Input: part model. Units: mm. Frame: model coordinates. Round coordinates to 2 decimals unless told otherwise and drop trailing zeros. Order: outer loops, then holes, each group sorted by start corner. A loop starts at its lowest first (then second) coordinate and runs counter-clockwise, first axis right, second up. Notation, with made-up numbers: (19.5, -2.75) -> (26.5, -2.75) arc R21 cw to (26.5, 26.25) -> close; hole circle Ø5 at (40, 72). An arc over 180 degrees is marked (long way). Use a Markdown table: item, result.
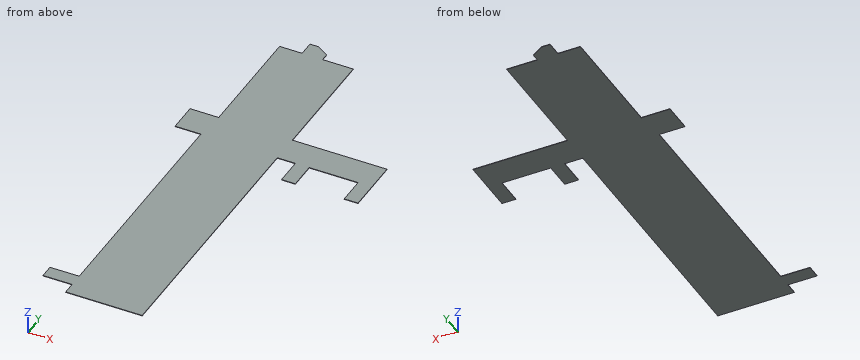
from build123d import *

# Parameters (mm, degrees)
SKETCH_1_W      = 16
SKETCH_1_H      = 30
SKETCH_1_W_2    = 27
SKETCH_1_H_2    = 53
SKETCH_1_W_3    = 60
SKETCH_1_H_3    = 55
SKETCH_1_H_4    = 57.5
SKETCH_1_H_5    = 117
SKETCH_1_H_6    = 117.5
SKETCH_1_W_4    = 125.5
SKETCH_1_H_7    = 60.4
SKETCH_1_H_8    = 230.9
EXTRUDE_1_DEPTH = 1
SKETCH_2_W      = 16
SKETCH_2_H      = 30
EXTRUDE_2_DEPTH = 10


with BuildPart() as part:
    # 草图1 → 拉伸1 (new body)
    with BuildSketch(Plane.XY.offset(42)):
        with Locations((450.5, -369.2)):
            Rectangle(SKETCH_1_W, SKETCH_1_H)
        Polygon((384.5, -354.2), (384.5, -384.2), (398.5, -384.2), (400.5, -384.2), (400.5, -354.2), align=None)
        with Locations((714, -700.1)):
            Rectangle(SKETCH_1_W_2, SKETCH_1_H_2)
        with Locations((591.5, -700.1)):
            Rectangle(SKETCH_1_W_2, SKETCH_1_H_2)
        Polygon((501.5, -423.1), (482.5, -423.1), (482.5, -443.7), (542.5, -443.7), (542.5, -413.6), (501.5, -413.6), align=None)
        Polygon((482.5, -410.1), (501.5, -410.1), (501.5, -413.6), (542.5, -413.6), (542.5, -384.2), (482.5, -384.2), align=None)
        with Locations((512.5, -471.2)):
            Rectangle(SKETCH_1_W_3, SKETCH_1_H_3)
        with Locations((428.5, -470.45)):
            Rectangle(SKETCH_1_W_3, SKETCH_1_H_4)
        Polygon((398.5, -384.2), (400.5, -384.2), (442.5, -384.2), (458.5, -384.2), (458.5, -441.7), (398.5, -441.7), align=None)
        with Locations((428.5, -557.7)):
            Rectangle(SKETCH_1_W_3, SKETCH_1_H_5)
        with Locations((512.5, -557.45)):
            Rectangle(SKETCH_1_W_3, SKETCH_1_H_6)
        with Locations((479.75, -1157.9)):
            Rectangle(SKETCH_1_W_4, SKETCH_1_H_7)
        Polygon((417, -896.8), (542.5, -896.8), (542.5, -786.2), (417.295919732, -786.2), align=None)
        Polygon((417.295919732, -786.2), (417.598084778, -673.265814274), (393, -673.2), (393, -1136.7), (336, -1137.1), (336, -1163.6), (393, -1163.6), (393, -1188.1), (417, -1188.1), (417, -1127.7), (417, -896.8), align=None)
        Polygon((542.5, -786.2), (542.5, -673.6), (417.598084778, -673.265814274), (417.295919732, -786.2), align=None)
        with Locations((479.75, -1012.25)):
            Rectangle(SKETCH_1_W_4, SKETCH_1_H_8)
        Polygon((393, -673.2), (342.5, -673.2), (342.5, -616.2), (398.5, -616.2), (458.5, -616.2), (458.5, -499.2), (458.5, -441.7), (458.5, -384.2), (458.5, -354.2), (482.5, -369.2), (482.5, -384.2), (482.5, -410.1), (501.5, -410.1), (501.5, -413.6), (501.5, -423.1), (482.5, -423.1), (482.5, -443.7), (482.5, -498.7), (482.5, -616.2), (542.5, -616.2), (727.5, -616.2), (727.5, -673.6), (700.5, -673.6), (605, -673.6), (578, -673.6), (542.5, -673.6), (417.598084778, -673.265814274), align=None)
    extrude(amount=-EXTRUDE_1_DEPTH)

    # 草图2 → 拉伸2 (cut)
    with BuildSketch(Plane.XY.offset(42)):
        with Locations((392.5, -369.2)):
            Rectangle(SKETCH_2_W, SKETCH_2_H)
    extrude(amount=-EXTRUDE_2_DEPTH, mode=Mode.SUBTRACT)


solid = part.part
1) Cut plane B-B on y = -1043.5. Return loops of the section in (x, z).
Answer key:
| item | result |
|---|---|
| outline | (393, 41) -> (542.5, 41) -> (542.5, 42) -> (393, 42) -> close |
2) Ray query, probe 1 along X at (y, z) = (-705, 41.35); probe 2 along Y at (x, z) = (374.5, 41.85); probe 3 along Y at (x, z) = (499, 41.7). Return the intervals inside material, ascending.
Answer key:
| item | result |
|---|---|
| probe 1 | x = 393 to 542.5, 578 to 605, 700.5 to 727.5 |
| probe 2 | y = -1163.6 to -1136.83, -673.2 to -616.2 |
| probe 3 | y = -1188.1 to -384.2 |
3) Contact query for flat-ended pins moving along their axis: P1, Ø0.5, axis at x = 717.5, z = 41.5, coming from the -Y side; P2, Ø0.5, axis at y = -636.5, z = 41.5, coming from the -X side; P3, Ø0.5, axis at y = -913, z = 41.5, coming from the -X side. Output: stop coordinate, or through.
Answer key:
| item | result |
|---|---|
| P1 | stops at y = -726.6 |
| P2 | stops at x = 342.5 |
| P3 | stops at x = 393 |
4) Cut plane C-C on x = 420. Return loops of the section in (y, z).
Answer key:
| item | result |
|---|---|
| outline | (-1188.1, 41) -> (-384.2, 41) -> (-384.2, 42) -> (-1188.1, 42) -> close |
5) Cut plane A-A on z = 41.6. Return loops of the section in (x, y), and give its area (3 significant figures).
Answer key:
| item | result |
|---|---|
| outline | (336, -1163.6) -> (393, -1163.6) -> (393, -1188.1) -> (542.5, -1188.1) -> (542.5, -673.6) -> (578, -673.6) -> (578, -726.6) -> (605, -726.6) -> (605, -673.6) -> (700.5, -673.6) -> (700.5, -726.6) -> (727.5, -726.6) -> (727.5, -616.2) -> (542.5, -616.2) -> (542.5, -384.2) -> (482.5, -384.2) -> (482.5, -369.2) -> (458.5, -354.2) -> (442.5, -354.2) -> (442.5, -384.2) -> (398.5, -384.2) -> (398.5, -616.2) -> (342.5, -616.2) -> (342.5, -673.2) -> (393, -673.2) -> (393, -1136.7) -> (336, -1137.1) -> close |
| area | 138,000 mm^2 |
